from build123d import *

# Parameters (mm, degrees)
SALIENTE_EXTRUIR1_DEPTH = 3.3


with BuildPart() as part:
    # Croquis1 → Saliente-Extruir1 (new body)
    with BuildSketch(Plane.XY):
        with BuildLine():
            Line((-0.15, -6.133444496), (-0.15, -9.433444496))
            Line((-0.15, -9.433444496), (-0.15, -11.04132323))
            Line((-0.15, -11.04132323), (-2.35, -11.04132323))
            Line((-2.35, -11.04132323), (-2.35, -9.433444496))
            Line((-2.35, -9.433444496), (-2, -9.433444496))
            Line((-2, -9.433444496), (-2, 1.070879644))
            Line((-2, 1.070879644), (-3.65, 1.070879644))
            ThreePointArc((-3.65, 1.070879644), (0, 4.720879644), (3.65, 1.070879644))
            Line((3.65, 1.070879644), (2, 1.070879644))
            Line((2, 1.070879644), (2, -9.433444496))
            Line((2, -9.433444496), (2.35, -9.433444496))
            Line((2.35, -9.433444496), (2.35, -11.04132323))
            Line((2.35, -11.04132323), (0.15, -11.04132323))
            Line((0.15, -11.04132323), (0.15, -9.433444496))
            Line((0.15, -9.433444496), (0.15, -6.133444496))
            ThreePointArc((0.15, -6.133444496), (0, -5.156474895), (-0.15, -6.133444496))
        make_face()
    extrude(amount=SALIENTE_EXTRUIR1_DEPTH)


solid = part.part
Geometry: final body of the model. Coordinates: model frame, mm. A direction names the side the tool comes from. Round coordinates to 2 decimals unless told otherwise and drop trailing zeros. Loops run counter-clockwise (first coordinate to the right, second up) from the corner with the lowest first, then second, coordinate; pieces in that order, holes last. Notation, with made-up numbers: M 31,4 L 43,4 A16 ccw 43,27 Z; hole C 24,-4.5 d3. An arc over 180 degrees is marked long. One line per question, with ' | ' between items.
(1) Cut plane C-C on y = -1.75. Return the cut outline in (x, z).
Check result:
outline: M -2,0 L 2,0 L 2,3.3 L -2,3.3 Z
(2) Pull-direction query (Y, two-part tool) for faces 6 (the flat face through (1, -11.041, 2)), 7 (the cylindrical face through (-0.08, 4.72, 1.63)), 8 (the flat face through (3, 1.071, 2)), 9 (the flat face through (-2, -4, 2)); classes: +Y half, -Y half, draft (parallel to the pull), parting line (faces both ways), or undercut.
Check result:
face 6: -Y half | face 7: +Y half | face 8: undercut | face 9: undercut
(3) Cut plane D-D on x = 0. Return the cut outline in (y, z).
Check result:
outline: M -5.16,0 L 4.72,0 L 4.72,3.3 L -5.16,3.3 Z
(4) Cut plane B-B on z = 2.1. Return the cut outline in (x, y), plus the area to 3 significant figures.
Check result:
outline: M -3.65,1.07 L -2,1.07 L -2,-9.43 L -2.35,-9.43 L -2.35,-11.04 L -0.15,-11.04 L -0.15,-6.13 A0.5 cw long 0.15,-6.13 L 0.15,-11.04 L 2.35,-11.04 L 2.35,-9.43 L 2,-9.43 L 2,1.07 L 3.65,1.07 A3.65 ccw Z | area: 68.2 mm2
(5) Cut plane A-A on y = -8.25. Return the cut outline in (x, z).
Check result:
outline: M -2,0 L -0.15,0 L -0.15,3.3 L -2,3.3 Z; M 0.15,0 L 2,0 L 2,3.3 L 0.15,3.3 Z
(6) Contact query for flat-ended pins moving along their axis: P1, Ø0.5, axis at y = -10, z = 1, coming from the -X side; P2, Ø1.8, axis at y = -10, z = 2.5, coming from the +X side; P3, Ø1, axis at y = -4, z = 1.5, coming from the +X side. Output: stop coordinate, or through.
Check result:
P1: stops at x = -2.35 | P2: stops at x = 2.35 | P3: stops at x = 2
(7) Access query for faces 1 (the flat face through (-2.35, -10, 2)), 2 (the flat face through (2.35, -10, 2)), 3 (the flat face through (-3, 1.071, 2)), 4 (the flat face through (2, -4, 2)), 5 (the flat face through (-0.15, -9, 2)). Directions: +Z, -Z, +X, -X, +Y, -Y. A direction counts if a zero-diameter tool reaches every point of the face in a straight line with its end or side. Return the directions, or none.
Check result:
face 1: +Z, -Z, -X, -Y | face 2: +Z, -Z, +X, -Y | face 3: +Z, -Z, -X | face 4: +Z, -Z, +X | face 5: +Z, -Z, -Y
(8) Material intervals for line 1 along X through (y, z) = (-8, 2.6); line 2 along X through (y, z) = (-9.75, 1.75); line 3 along X through (y, z) = (-3, 0.35), sorted ascending. Write a range as from..to.
Check result:
line 1: x = -2..-0.15, 0.15..2 | line 2: x = -2.35..-0.15, 0.15..2.35 | line 3: x = -2..2
